Check sheet for the modelled part. Datum: model origin and axes. Units: mm. Face numbers are marked on the shaded views. A direction names the side the tool comes from. Round coordinates to 2 decimals unless told otherwise and drop trailing zeros. Order: outer loops, then holes, each group sorted by start corner. A loop starts at its lowest first (then second) coordinate and runs counter-clockwise, first axis right, second up.
Q1. Cross-section at C-C on z = 0. Record the cut outline in (x, y), then the cut area to 3 significant figures.
Q2. Mould release check, pull along Z, two halves, no side actions. Record for the marked faces 1, 2, 3 and 4: +Z half, -Z half, draft (parallel to the pull), parting line (faces both ways), or undercut.
Q3. Cross-section at A-A on x = -29. Record the cut outline in (y, z) (3 decimals).
Q4. Scan lines: probe 1 along X at (y, z) = (5.75, 11.5) (3 decimals); probe 2 along X at (y, z) = (3, -11.5) (3 decimals); probe 3 along Z at (x, y) = (-28.5, 7). Record each from-to range of solid material in increasing order.
Q5. Set-up check for the marked faces 5, 6 and 7: record each of +Z, -Z, +X, -X, +Y, -Y from which the full face is reachable in a straight line by a thin tool's end or side.
Q6. Cross-section at D-D on y = -14.25. Record the cut outline in (x, z) (3 decimals), then the cut area to 3 significant figures.
Q7. Depth check by flat-ended pin: P1, Ø1.2, axis at x = 30.5, y = 2, coming from the -Z side; P2, Ø5, axis at x = -15.5, y = 2.5, coming from the -Z side; P3, Ø3, axis at x = -31.5, y = 2, coming from the +Z side. Enter the tip coordinate at first touch or a pass-through.
Q8. Cross-section at B-B on z = 23.6. Record the cut outline in (x, y) (3 decimals), then the cut area to 4 significant figures.
from build123d import *

# Parameters (mm, degrees)
SKETCH1_R                  = 1.375
MOUNT_PLATE_DEPTH          = 4
FEUSELAGE_MOUNT_DEPTH      = 8
SKETCH8_R                  = 3.5
SKETCH8_R_2                = 1.375
MOUNTING_HOLES_DEPTH       = 5
FASTENING_HOLES_DEPTH      = 54.661625022
FASTENING_HOLES_DEPTH_BACK = 8
SKETCH10_R                 = 2.525
FILLET1_R                  = 5


with BuildPart() as part:
    # Sketch1 → Mount_Plate (new body)
    with BuildSketch(Plane(origin=(0, 0, 0), x_dir=(1, 0, 0), z_dir=(0, 1, 0))):
        Polygon((37.5, 20), (37.5, 9), (33.5, 5), (33.5, -5), (37.5, -9), (37.5, -20), (27, -20), (15, -8), (-15, -8), (-27, -20), (-37.5, -20), (-37.5, -9), (-33.5, -5), (-33.5, 5), (-37.5, 9), (-37.5, 20), (-27, 20), (-15, 8), (15, 8), (27, 20), align=None)
        with Locations(Location((-29, -11.5, 0), (0, 0, 270))):
            Circle(SKETCH1_R, mode=Mode.SUBTRACT)
        with Locations(Location((-29, 11.5, 0), (0, 0, 90))):
            Circle(SKETCH1_R, mode=Mode.SUBTRACT)
        with Locations(Location((29, -11.5, 0), (0, 0, 90))):
            Circle(SKETCH1_R, mode=Mode.SUBTRACT)
        with Locations(Location((29, 11.5, 0), (0, 0, 270))):
            Circle(SKETCH1_R, mode=Mode.SUBTRACT)
    extrude(amount=MOUNT_PLATE_DEPTH)

    # Sketch4 → Feuselage_Mount (add, symmetric)
    with BuildSketch(Plane(origin=(0, 0, 0), x_dir=(0, 0, -1), z_dir=(1, 0, 0))):
        with BuildLine():
            Line((-16.6, -9.6), (-28.6, -9.6))
            Line((-28.6, -9.6), (-28.6, -16.6))
            Line((-28.6, -16.6), (-12.6, -16.6))
            ThreePointArc((-12.6, -16.6), (0, -4), (12.6, -16.6))
            Line((12.6, -16.6), (28.6, -16.6))
            Line((28.6, -16.6), (28.6, -9.6))
            Line((28.6, -9.6), (16.6, -9.6))
            Line((16.6, -9.6), (8, 0))
            Line((8, 0), (-8, 0))
            Line((-8, 0), (-16.6, -9.6))
        make_face()
    extrude(amount=FEUSELAGE_MOUNT_DEPTH, both=True)

    # Sketch8 → Mounting_Holes (add)
    # profile 1 of 4: a face of its own
    with BuildSketch(Plane(origin=(0, 4, 0), x_dir=(1, 0, 0), z_dir=(0, 1, 0))):
        with Locations(Location((29, -11.5, 0), (0, 0, 90))):
            Circle(SKETCH8_R)
        with Locations(Location((29, -11.5, 0), (0, 0, 90))):
            Circle(SKETCH8_R_2, mode=Mode.SUBTRACT)
    # profile 2 of 4: a face of its own
    with BuildSketch(Plane(origin=(0, 4, 0), x_dir=(1, 0, 0), z_dir=(0, 1, 0))):
        with Locations(Location((-29, 11.5, 0), (0, 0, 90))):
            Circle(SKETCH8_R)
        with Locations(Location((-29, 11.5, 0), (0, 0, 90))):
            Circle(SKETCH8_R_2, mode=Mode.SUBTRACT)
    # profile 3 of 4: a face of its own
    with BuildSketch(Plane(origin=(0, 4, 0), x_dir=(1, 0, 0), z_dir=(0, 1, 0))):
        with Locations(Location((-29, -11.5, 0), (0, 0, 90))):
            Circle(SKETCH8_R)
        with Locations(Location((-29, -11.5, 0), (0, 0, 270))):
            Circle(SKETCH8_R_2, mode=Mode.SUBTRACT)
    # profile 4 of 4: a face of its own
    with BuildSketch(Plane(origin=(0, 4, 0), x_dir=(1, 0, 0), z_dir=(0, 1, 0))):
        with Locations(Location((29, 11.5, 0), (0, 0, 90))):
            Circle(SKETCH8_R)
        with Locations(Location((29, 11.5, 0), (0, 0, 270))):
            Circle(SKETCH8_R_2, mode=Mode.SUBTRACT)
    extrude(amount=MOUNTING_HOLES_DEPTH)

    # Sketch10 → Fastening_Holes (cut, two sides: drawn at the far end of the back side and taken through both)
    with BuildSketch(Plane.XZ.offset(16.6).offset(-FASTENING_HOLES_DEPTH_BACK)):
        with Locations(Location((0, 23.6, 0), (0, 0, 90))):
            Circle(SKETCH10_R)
        with Locations(Location((0, -23.6, 0), (0, 0, 90))):
            Circle(SKETCH10_R)
    extrude(amount=FASTENING_HOLES_DEPTH + FASTENING_HOLES_DEPTH_BACK, mode=Mode.SUBTRACT)

    # Fillet1
    fillet1_edges = [part.edges().sort_by_distance(p)[0] for p in [
        (0, 0, 8),
        (0, -9.6, 16.6),
        (0, -9.6, -16.6),
        (0, 0, -8),
    ]]
    fillet(fillet1_edges, radius=FILLET1_R)


solid = part.part
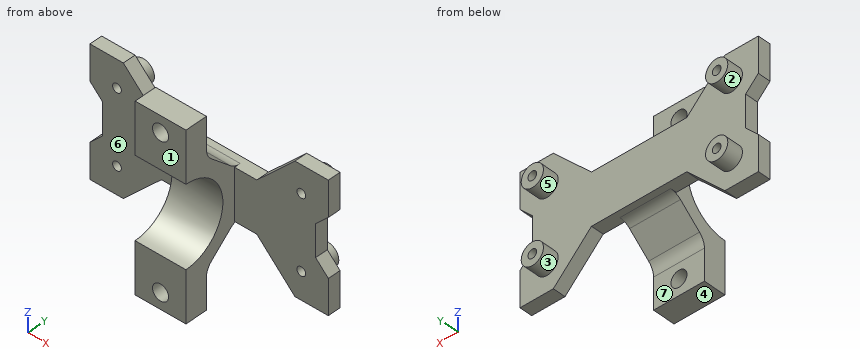
Results found:
1. outline: (-33.5, 0) - (-8, 0) - (-8, -4) - (8, -4) - (8, 0) - (33.5, 0) - (33.5, 4) - (-33.5, 4) - close
1. area: 332 mm2
2. face 1: draft
2. face 2: undercut
2. face 3: undercut
2. face 4: -Z half
3. outline: (0, -20) - (4, -20) - (4, -15) - (9, -15) - (9, -12.875) - (0, -12.875) - close; (0, -10.125) - (9, -10.125) - (9, -8) - (4, -8) - (4, 8) - (9, 8) - (9, 10.125) - (0, 10.125) - close; (0, 12.875) - (9, 12.875) - (9, 15) - (4, 15) - (4, 20) - (0, 20) - close
4. probe 1: x = -32.5 to -30.375, -27.625 to -25.5, 25.5 to 27.625, 30.375 to 32.5
4. probe 2: x = -37.5 to -30.375, -27.625 to -18.5, 18.5 to 27.625, 30.375 to 37.5
4. probe 3: z = -14.96 to -12.78, -10.22 to -8.04, 8.04 to 10.22, 12.78 to 14.96
5. face 5: +Y
5. face 6: +Z, -Z, -X, -Y
5. face 7: -Z, +X, -X, +Y
6. outline: (-8, -28.6) - (8, -28.6) - (8, -12.379) - (-8, -12.379) - close; (-8, 12.379) - (8, 12.379) - (8, 28.6) - (-8, 28.6) - close; hole circle Ø5.05 at (0, -23.6); hole circle Ø5.05 at (0, 23.6)
6. area: 479 mm2
7. P1: stops at z = -20
7. P2: stops at z = -11
7. P3: stops at z = 20
8. outline: (-8, -16.6) - (-2.525, -16.6) - (-2.525, -9.6) - (-8, -9.6) - close; (2.525, -16.6) - (8, -16.6) - (8, -9.6) - (2.525, -9.6) - close
8. area: 76.65 mm2
